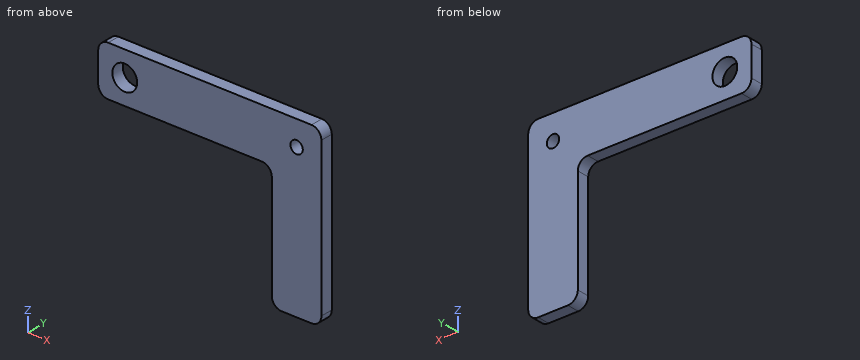
from build123d import *

# Parameters (mm, degrees)
F0_R     = 3.175
F1_DEPTH = 6.35
F2_R     = 5.08
F3_R     = 6.35
F4_DEPTH = 25.4


with BuildPart() as f1:
    # F0 (on Front) → F1 (new body)
    with BuildSketch(Plane.XZ):
        Polygon((88.9, 63.5), (88.9, 0), (114.3, 0), (114.3, 88.9), (0, 88.9), (0, 63.5), align=None)
        with Locations((101.6, 76.2)):
            Circle(F0_R, mode=Mode.SUBTRACT)
    extrude(amount=F1_DEPTH)

    # F2
    f2_edges = [f1.edges().sort_by_distance(p)[0] for p in [
        (0, -3.175, 63.5),
        (0, -3.175, 88.9),
        (114.3, -3.175, 88.9),
        (114.3, -3.175, 0),
        (88.9, -3.175, 0),
        (88.9, -3.175, 63.5),
    ]]
    fillet(f2_edges, radius=F2_R)

    # F3 (on face) → F4 (cut)
    with BuildSketch(Plane(origin=(0, 0, 0), x_dir=(-1, 0, 0), z_dir=(0, 1, 0))):
        with Locations((-13.5994189943, 76.2)):
            Circle(F3_R)
    extrude(amount=-F4_DEPTH, mode=Mode.SUBTRACT)


solid = f1.part
Check sheet for the modelled part. Datum: model origin and axes. Units: mm. Coordinates: 2 decimals unless noted, no trailing zeros. Loops run counter-clockwise (first coordinate to the right, second up) from the corner with the lowest first, then second, coordinate; pieces in that order, holes last. Notation, with made-up numbers: (-36.5, -32.75) -> (13.5, -32.75) arc R17 ccw to (13.5, -18.75) -> close; hole circle Ø2 at (30.5, 77.25). An arc over 180 degrees is marked (long way). Answer in a Markdown table with one row per item.
1. Sectioned sample at D-D, the plane x = 55. Record the boundary of the cut face in (y, z), then the cut area to 3 significant figures.
Check values:
| item | result |
|---|---|
| outline | (-6.35, 63.5) -> (0, 63.5) -> (0, 88.9) -> (-6.35, 88.9) -> close |
| area | 161 mm2 |
2. Material ranges on line 1 along X through (y, z) = (-0.5, 76); line 2 along Z through (x, y) = (61.5, -4); line 3 along X through (y, z) = (-1.25, 23), recorded low to high. Write a range as [from, to].
Check values:
| item | result |
|---|---|
| line 1 | x = [0, 7.25], [19.95, 98.43], [104.77, 114.3] |
| line 2 | z = [63.5, 88.9] |
| line 3 | x = [88.9, 114.3] |
3. Sectioned sample at B-B, the plane x = 101.6. Record the boundary of the cut face in (y, z) (3 decimals).
Check values:
| item | result |
|---|---|
| outline | (-6.35, 0) -> (0, 0) -> (0, 73.025) -> (-6.35, 73.025) -> close; (-6.35, 79.375) -> (0, 79.375) -> (0, 88.9) -> (-6.35, 88.9) -> close |
4. Go/stop test with flat-tipped pins: pin 1 (11.5 mm diameter, centred on x = 13.6, z = 76.2, fed in from -Y); pin 2 (1.9 mm diameter, centred on y = -3, z = 42.5, fed in from -X). Record where each tip stops, or that it passes through.
Check values:
| item | result |
|---|---|
| pin 1 | passes through |
| pin 2 | stops at x = 88.9 |
5. Sectioned sample at A-A, the plane z = 76.2. Record the boundary of the cut face in (x, y) (3 decimals), then the cut area to 3 significant figures.
Check values:
| item | result |
|---|---|
| outline | (0, -6.35) -> (7.249, -6.35) -> (7.249, 0) -> (0, 0) -> close; (19.949, -6.35) -> (98.425, -6.35) -> (98.425, 0) -> (19.949, 0) -> close; (104.775, -6.35) -> (114.3, -6.35) -> (114.3, 0) -> (104.775, 0) -> close |
| area | 605 mm2 |
6. Sectioned sample at C-C, the plane y = -1. Record the boundary of the cut face in (x, z) (3 decimals).
Check values:
| item | result |
|---|---|
| outline | (0, 68.58) arc R5.08 ccw to (5.08, 63.5) -> (83.82, 63.5) arc R5.08 cw to (88.9, 58.42) -> (88.9, 5.08) arc R5.08 ccw to (93.98, 0) -> (109.22, 0) arc R5.08 ccw to (114.3, 5.08) -> (114.3, 83.82) arc R5.08 ccw to (109.22, 88.9) -> (5.08, 88.9) arc R5.08 ccw to (0, 83.82) -> close; hole circle Ø12.7 at (13.599, 76.2); hole circle Ø6.35 at (101.6, 76.2) |
